Geometry check sheet. Reference: the model listing, model coordinates, mm. A direction names the side the tool comes from. Coordinates: 2 decimals unless noted, no trailing zeros. Write each loop counter-clockwise with the first axis right and the second up, starting at its lowest first coordinate (ties: lowest second). Pieces come first, ordered by that corner, then holes. Notation, with made-up numbers: (68, 16) -> (118, 16) arc R27 ccw to (118, 36) -> close; hole circle Ø9 at (-23.75, -15). An arc over 180 degrees is marked (long way). Answer in a Markdown table with one row per item. Add a question column.
1. Depth check by flat-ended pin: P1, Ø6, axis at y = 43, z = -1.5, coming from the -X side; P2, Ø8.5, axis at x = -4.5, y = 14, coming from the +Z side; P3, Ø0.9, axis at x = -2, z = -7.5, coming from the -Y side; P4, Ø3.5, axis at x = 3.5, z = -7, coming from the -Y side. Enter the tip coordinate at first touch or a pass-through.
2. Set-up check for faces 4 (the flat face through (-7, -3, -7)), 5 (the flat face through (-8.5, 1, -8)), 6 (the flat face through (-3, 1, -8)): record each of +Z, -Z, +X, -X, +Y, -Y from which the full face is reachable in a straight line by a thin tool's end or side.
3. Cross-section at B-B on y = 46. Record the cut outline in (x, z).
4. Mould release check, pull along Y, two halves, no side actions. Record for faces 1 (the cylindrical face through (1.77, -14.1, 2.14)), 2 (the cylindrical face through (1.77, 71.14, 2.1)), 3 (the flat face through (-4, 15, -8)): pulls with the +Y half, pulls with the -Y half, needs draft (parallel to the pull), parting line crosses it, or undercut.
5. Cross-section at A-A on y = -5.5. Record the cut outline in (x, z).
6. Scan lines: L1, parallel to X at y = 34.5, z = -1.25; L2, parallel to Z at x = -0.5, y = 43.5; L3, parallel to X at y = 9, z = -6.75. Record each from-to range of solid material in increasing order. Write a range as from..to.
```python
from build123d import *

# Parameters (mm, degrees)
EXTRUDE_1_DEPTH             = 3
SKETCH_2_W                  = 3
SKETCH_2_H                  = 72.000001073
EXTRUDE_2_DEPTH             = 1.5
CUT_EXTRUDE_1_DEPTH         = 73.753007862
SKETCH_4_W                  = 1.5
SKETCH_4_H                  = 69.000001073
CUT_EXTRUDE_2_DEPTH         = 73.753007862
EXTRUDE_3_DEPTH             = 3
DRAFT_1_ANGLE               = 45
HOLE_WIZARD_2_7_2_7_1_D     = 3.5
HOLE_WIZARD_2_7_2_7_1_DEPTH = 5.000000075
FILLET_1_R                  = 3
CHAMFER_1_SIZE              = 2.000001073
CHAMFER_1_SIZE2             = 2
CHAMFER_2_SIZE              = 2
CHAMFER_2_SIZE2             = 2.000001073
CHAMFER_4_SIZE              = 0.5


with BuildPart() as part:
    # ｽｹｯﾁ1 → ﾎﾞｽ - 押し出し1 (new body)
    with BuildSketch(Plane.XY.offset(-6)):
        with BuildLine():
            Line((5.000000075, 72.00000107), (-6.999999925, 72.00000107))
            Line((-6.999999925, 72.00000107), (-6.999999925, -7))
            ThreePointArc((-6.999999925, -7), (-9.999999925, -10), (-6.999999925, -13))
            Line((-6.999999925, -13), (5.000000075, -13))
            Line((5.000000075, -13), (5.000000075, 72.00000107))
        make_face()
    extrude(amount=-EXTRUDE_1_DEPTH)

    # ｽｹｯﾁ2 → ﾎﾞｽ - 押し出し2 (add)
    with BuildSketch(Plane.ZY.offset(6.999999925)):
        with Locations((-7.5, 36.000000537)):
            Rectangle(SKETCH_2_W, SKETCH_2_H)
    extrude(amount=EXTRUDE_2_DEPTH)

    # ｽｹｯﾁ3 → ｶｯﾄ - 押し出し1 (cut, through all)
    with BuildSketch(Plane(origin=(0, 0, -9), x_dir=(-1, 0, 0), z_dir=(0, 0, -1))):
        Polygon((3, -13), (3, 15), (4.5, 15), (4.5, 17), (0, 17), (0, -13), align=None)
    extrude(amount=-CUT_EXTRUDE_1_DEPTH, mode=Mode.SUBTRACT)

    # ｽｹｯﾁ4 → ｶｯﾄ - 押し出し2 (cut, through all)
    with BuildSketch(Plane.XY.offset(-6)):
        with Locations((-7.749999925, 37.500000537)):
            Rectangle(SKETCH_4_W, SKETCH_4_H)
    extrude(amount=-CUT_EXTRUDE_2_DEPTH, mode=Mode.SUBTRACT)

    # ｽｹｯﾁ5 → ﾎﾞｽ - 押し出し3 (add)
    with BuildSketch(Plane(origin=(0, 0, 0), x_dir=(0, -1, 0), z_dir=(-1, 0, 0))):
        Polygon((-72.000001073, 3), (-72.000001073, -3), (-72.000001073, -6), (14.999998927, -6), (14.999998927, 3), align=None)
    extrude(amount=-EXTRUDE_3_DEPTH)

    # 抜き勾配1
    draft_1_faces = [part.faces().sort_by_distance(p)[0] for p in [
        (-7.749999925, 3, -7.5),
    ]]
    draft(draft_1_faces, Plane(origin=(-6.999999925, 3, -9), x_dir=(0, -1, 0), z_dir=(-1, 0, 0)), DRAFT_1_ANGLE)

    # Ø2.7 (2.7) 直径の穴1
    with Locations(Plane.ZY):
        with Locations((0, 69.000001073), (0, -11.999998927)):
            Hole(HOLE_WIZARD_2_7_2_7_1_D / 2, depth=HOLE_WIZARD_2_7_2_7_1_DEPTH)

    # ﾌｨﾚｯﾄ1
    fillet_1_edges = [part.edges().sort_by_distance(p)[0] for p in [
        (1.5, 72.000001073, 3),
        (1.5, -14.999998927, 3),
    ]]
    fillet(fillet_1_edges, radius=FILLET_1_R)

    # 面取り1
    chamfer_1_edges = [part.edges().sort_by_distance(p)[0] for p in [
        (-6.999999925, 72.000001073, -7.5),
    ]]
    chamfer_1_side = [part.faces().sort_by_distance(p)[0] for p in [
        (1.5, 72.00000107, -0.15),
    ]]
    chamfer(chamfer_1_edges, length=CHAMFER_1_SIZE, length2=CHAMFER_1_SIZE2, reference=chamfer_1_side[0])

    # 面取り2
    chamfer_2_edges = [part.edges().sort_by_distance(p)[0] for p in [
        (5.000000075, 72.00000107, -7.5),
    ]]
    chamfer_2_side = [part.faces().sort_by_distance(p)[0] for p in [
        (0.56250042, 72.00000107, -5.812499887),
    ]]
    chamfer(chamfer_2_edges, length=CHAMFER_2_SIZE, length2=CHAMFER_2_SIZE2, reference=chamfer_2_side[0])

    # 面取り4
    chamfer_4_edges = [part.edges().sort_by_distance(p)[0] for p in [
        (0, -14.999998927, -3),
        (0, 28.500001071, 3),
        (0, 72.000001073, -3),
        (0, -14.121319271, 2.121320344),
        (0, 71.121321414, 2.121320344),
    ]]
    chamfer(chamfer_4_edges, length=CHAMFER_4_SIZE)


solid = part.part
```
Results found:
| question | item | result |
|---|---|---|
| 1 | P1 | stops at x = 0 |
| 1 | P2 | stops at z = -6 |
| 1 | P3 | stops at y = 17 |
| 1 | P4 | stops at y = -15 |
| 2 | face 4 | +Z, -Z, -X |
| 2 | face 5 | +Z, -Z, -X, +Y |
| 2 | face 6 | +Z, -Z, -Y |
| 3 | outline | (-7, -9) -> (5, -9) -> (5, -6) -> (3, -6) -> (3, 3) -> (0.5, 3) -> (0, 2.5) -> (0, -6) -> (-7, -6) -> close |
| 4 | face 1 | pulls with the -Y half |
| 4 | face 2 | pulls with the +Y half |
| 4 | face 3 | undercut |
| 5 | outline | (-7, -9) -> (-3, -9) -> (-3, -6) -> (-7, -6) -> close; (0, -9) -> (5, -9) -> (5, -6) -> (3, -6) -> (3, 3) -> (0.5, 3) -> (0, 2.5) -> close |
| 6 | L1 | x = 0..3 |
| 6 | L2 | z = -9..-6 |
| 6 | L3 | x = -7..-3, 0..5 |
